```python
from build123d import *


with BuildPart() as part:
    # Austragung1: sweep along a path in Skizze2
    with BuildLine(Plane.XY) as austragung1_path:
        Line((-2020, 217), (0, 217))
        ThreePointArc((0, 217), (38.99906336, 177.729709462), (-0.540568093, 139.003746512))
        Line((-0.540568093, 139.003746512), (-2020.346518009, 167.00240161))
        ThreePointArc((-2020.346518009, 167.00240161), (-2044.99939959, 192.173263165), (-2020, 217))
    # Skizze3 → Austragung1 (sweep)
    with BuildSketch(Plane(origin=(0, 0, 0), x_dir=(0, 0, -1), z_dir=(1, 0, 0))):
        Polygon((202.5, 219), (-202.5, 219), (-202.5, 217), (0, 217), (202.5, 217), align=None)
    sweep(path=austragung1_path.line)


solid = part.part
```
Check sheet for the modelled part. Datum: model origin and axes. Units: mm. A direction names the side the tool comes from. Round coordinates to 2 decimals unless told otherwise and drop trailing zeros. Order: outer loops, then holes, each group sorted by start corner. A loop starts at its lowest first (then second) coordinate and runs counter-clockwise, first axis right, second up. Notation, with made-up numbers: (-27.5, 89.5) -> (23.5, 89.5) arc R10 ccw to (23.5, 105.5) -> close; hole circle Ø10 at (-31, 86.25). An arc over 180 degrees is marked (long way). Use CSV: the item, a comma, the result in double quotes.
(1) Depth check by flat-ended pin: pin 1 (6 mm diameter, centred on y = 154, z = 79.5, fed in from +X); pin 2 (10 mm diameter, centred on y = 171, z = 93, fed in from +X); pin 3 (8 mm diameter, centred on x = -807, z = 149, fed in from -Y); pin 4 (12 mm diameter, centred on y = 195, z = 121.5, fed in from -X). Enter the tip coordinate at first touch or a pass-through.
Worked out:
pin 1,"x = 35.21"
pin 2,"x = 40.95"
pin 3,"y = 148.13"
pin 4,"x = -2047"
(2) Cross-section at B-B (y = 202). Record the boundary of the cut face in (x, z), and give its area (3 significant figures).
Worked out:
outline,"(-2045.08, -202.5) -> (-2042.91, -202.5) -> (-2042.91, 202.5) -> (-2045.08, 202.5) -> close; (30.74, -202.5) -> (33.24, -202.5) -> (33.24, 202.5) -> (30.74, 202.5) -> close"
area,"1,890 mm²"
(3) Draft check along Y on faces 3 (the face through (-996, 219, -3)), 4 (the face through (38.996, 178.591, -2.835)), 5 (the face through (-2047, 192, 3)). Enter one of: pulls with the +Y half, pulls with the -Y half, needs draft (parallel to the pull), parting line crosses it, or undercut.
Worked out:
face 3,"pulls with the +Y half"
face 4,"undercut"
face 5,"parting line crosses it"
(4) Tool access check on faces 1 (the face through (-998.1, 217.3, -202.5)), 2 (the face through (-2045, 192, -3)). Record the directions out of +Z, -Z, +X, -X, +Y, -Y that give a thin tool (end or side, any length) a straight path to the whole face; none if there is none.
Worked out:
face 1,"-Z, +X, -X, +Y, -Y"
face 2,"+Z, -Z"
(5) Cross-section at A-A (z = -142). Record the boundary of the cut face in (x, y), and give its area (3 significant figures).
Worked out:
outline,"(-2020.37, 165) -> (-0.57, 137) arc R41 ccw (long way) to (0, 219) -> (-2020, 219) arc R27 ccw to start; hole (-2020.35, 167) -> (-0.54, 139) arc R39 ccw (long way) to (0, 217) -> (-2020, 217) arc R25 ccw to start"
area,"8,500 mm²"
(6) Material ranges on line 1 along Y through (x, z) = (-288, -75); line 2 along Y through (x, z) = (-1049.5, -185); line 3 along X through (y, z) = (192.5, -185.5) (3 decimals), recorded low to high. Write a range as from..to.
Worked out:
line 1,"140.99..142.99, 217..219"
line 2,"151.54..153.54, 217..219"
line 3,"-2046.995..-2044.995, 36.204..38.35"
(7) Cross-section at C-C (x = -1470). Record the boundary of the cut face in (y, z), and give its area (3 significant figures).
Worked out:
outline,"(157.37, -202.5) -> (159.37, -202.5) -> (159.37, 202.5) -> (157.37, 202.5) -> close; (217, -202.5) -> (219, -202.5) -> (219, 202.5) -> (217, 202.5) -> close"
area,"1,620 mm²"
